from build123d import *

# Parameters (mm, degrees)
F1_DEPTH  = 6
F1_FACE_W = 6
F1_FACE_H = 7.6992507409
F3_W      = 0.3979424946
F3_H      = 0.4551622551


with BuildPart() as f1:
    # F0 (on Front) → F1 (new body)
    with BuildSketch(Plane.XZ):
        with BuildLine():
            ThreePointArc((3.7797707351, 10.0635894784), (1.9207958125, 10.5770054102), (0, 10.75))
            ThreePointArc((0, 10.75), (-1.9207958125, 10.5770054102), (-3.7797707351, 10.0635894784))
            Line((-3.7797707351, 10.0635894784), (-9.5399799449, 4.9549250904))
            ThreePointArc((-9.5399799449, 4.9549250904), (0, -10.75), (9.5399799449, 4.9549250904))
            Line((9.5399799449, 4.9549250904), (3.7797707351, 10.0635894784))
        make_face()
        with BuildLine():
            ThreePointArc((0, 8.75), (6.1871843354, 6.1871843354), (8.75, 0))
            ThreePointArc((8.75, 0), (-6.1871843354, -6.1871843354), (0, 8.75))
        make_face(mode=Mode.SUBTRACT)
    extrude(amount=F1_DEPTH)

    # F1_face (on face) → F4 section 0
    with BuildSketch(Plane(origin=(6.65987534, -3, 7.5092572844), x_dir=(0, 1, 0), z_dir=(0.663527473, 0, 0.7481519181))):
        Rectangle(F1_FACE_W, F1_FACE_H)
    # F3 (on offset) → F4 section 1
    with BuildSketch(Plane(origin=(10.641040178, 0, 11.9981687931), x_dir=(0.7481519181, 0, -0.663527473), z_dir=(0.663527473, 0, 0.7481519181))):
        with Locations((-3.1523916405, -2.7441481361)):
            Rectangle(F3_W, F3_H)
    loft()

    # F5: F1 across plane


with BuildPart() as f1_1:
    add(f1.part)
    add(f1.part.mirror(Plane.YZ))


solid = f1_1.part
Input: part model. Units: mm. Frame: model coordinates. Give positions to 0.01 mm unless a question says otherwise; leave off trailing zeros. Write each loop counter-clockwise with the first axis right and the second up, starting at its lowest first coordinate (ties: lowest second). Pieces come first, ordered by that corner, then holes. Notation, with made-up numbers: M -11.5,37 L -3.5,37 A15 cw -3.5,58 Z; hole C 58.25,-31 d6. An arc over 180 degrees is marked long. Write item = value, one per line. Start each with the question number.
1) Cut plane A-A on x = -2. Return the cut outline in (y, z).
2) Cut plane B-B on z = 1.5. Return the cut outline in (x, y), then the cut area to 3 significant figures.
3) First-contact query: pin 1 Ø1.5 at (y, z) = (-2.5, 5.5) entering from -X; pin 2 Ø1 at (y, z) = (-2.5, 3) entering from +X. Flat tips, straight axial feed; report the tip coordinate or a pass-through.
4) Draft query along X for faces 1 (the cylindrical face through (-0.308, -2.958, -10.746)), 2 (the flat face through (-1, 0, -9)). Return one class per face: +X half, -X half, draft (parallel to the pull), parting line (faces both ways), or undercut.
5) Material intervals for line 1 along Z through (x, y) = (0, -2.85); line 2 along X through (y, z) = (-2.75, 4.5), sorted ascending. Write a range as [from, to].
Solved:
q1.outline = M -6,-10.56 L 0,-10.56 L 0,-8.52 L -6,-8.52 Z; M -6,8.52 L 0,8.52 L 0,10.56 L -6,10.56 Z
q2.outline = M -10.64,-6 L -8.62,-6 L -8.62,0 L -10.64,0 Z; M 8.62,-6 L 10.64,-6 L 10.64,0 L 8.62,0 Z
q2.area = 24.3 mm2
q3.pin_1 = -9.64
q3.pin_2 = 10.46
q4.face_1 = parting line
q4.face_2 = draft
q5.line_1 = [-10.75, -8.75], [8.75, 10.75]
q5.line_2 = [-9.76, -7.5], [7.5, 9.76]
